from build123d import *

# Parameters (mm, degrees)
SKETCH_1_R          = 15
SKETCH_1_R_2        = 7
EXTRUDE_1_DEPTH     = 2
CUT_EXTRUDE_1_REACH = 23.307
SKETCH_2_R          = 1.1
SKETCH_3_R          = 0.95


with BuildPart() as part:
    # 草图1 → 凸台-拉伸1 (new body)
    with BuildSketch(Plane(origin=(0, 0, 0), x_dir=(1, 0, 0), z_dir=(0, 1, 0))):
        with Locations(Location((0, 0, 0), (0, 0, 270))):
            Circle(SKETCH_1_R)
        with Locations(Location((0, 0, 0), (0, 0, 270))):
            Circle(SKETCH_1_R_2, mode=Mode.SUBTRACT)
    extrude(amount=EXTRUDE_1_DEPTH)

    # 草图2 → 切除-拉伸1 (cut, up to next)
    with BuildSketch(Plane(origin=(0, 2, 0), x_dir=(1, 0, 0), z_dir=(0, 1, 0)), mode=Mode.PRIVATE) as cut_extrude_1_sk1:
        with Locations(Location((12.5, 0, 0), (0, 0, 270))):
            Circle(SKETCH_2_R)
    cut_extrude_1_tool1 = extrude(cut_extrude_1_sk1.sketch, amount=-CUT_EXTRUDE_1_REACH, mode=Mode.PRIVATE) & part.part
    # 草图2 → 切除-拉伸1 (cut, up to next)
    with BuildSketch(Plane(origin=(0, 2, 0), x_dir=(1, 0, 0), z_dir=(0, 1, 0)), mode=Mode.PRIVATE) as cut_extrude_1_sk2:
        with Locations(Location((0, -12.5, 0), (0, 0, 270))):
            Circle(SKETCH_2_R)
    cut_extrude_1_tool2 = extrude(cut_extrude_1_sk2.sketch, amount=-CUT_EXTRUDE_1_REACH, mode=Mode.PRIVATE) & part.part
    # 草图2 → 切除-拉伸1 (cut, up to next)
    with BuildSketch(Plane(origin=(0, 2, 0), x_dir=(1, 0, 0), z_dir=(0, 1, 0)), mode=Mode.PRIVATE) as cut_extrude_1_sk3:
        with Locations(Location((-12.5, 0, 0), (0, 0, 270))):
            Circle(SKETCH_2_R)
    cut_extrude_1_tool3 = extrude(cut_extrude_1_sk3.sketch, amount=-CUT_EXTRUDE_1_REACH, mode=Mode.PRIVATE) & part.part
    # 草图2 → 切除-拉伸1 (cut, up to next)
    with BuildSketch(Plane(origin=(0, 2, 0), x_dir=(1, 0, 0), z_dir=(0, 1, 0)), mode=Mode.PRIVATE) as cut_extrude_1_sk4:
        with Locations(Location((0, 12.5, 0), (0, 0, 270))):
            Circle(SKETCH_2_R)
    cut_extrude_1_tool4 = extrude(cut_extrude_1_sk4.sketch, amount=-CUT_EXTRUDE_1_REACH, mode=Mode.PRIVATE) & part.part
    add(cut_extrude_1_tool1.solids().sort_by_distance((12.5, 2, 0))[0], mode=Mode.SUBTRACT)
    add(cut_extrude_1_tool2.solids().sort_by_distance((0, 2, 12.5))[0], mode=Mode.SUBTRACT)
    add(cut_extrude_1_tool3.solids().sort_by_distance((-12.5, 2, 0))[0], mode=Mode.SUBTRACT)
    add(cut_extrude_1_tool4.solids().sort_by_distance((0, 2, -12.5))[0], mode=Mode.SUBTRACT)

    # 草图3 → 切除-旋转1 (revolve, cut)
    with BuildSketch(Plane.XY, mode=Mode.PRIVATE) as cut_revolve_1_sk:
        with Locations((9.05, 2)):
            Circle(SKETCH_3_R)
    revolve(cut_revolve_1_sk.sketch.rotate(Axis((0, 2, 0), (0, 1, 0)), 90), axis=Axis((0, 2, 0), (0, 1, 0)), mode=Mode.SUBTRACT)


solid = part.part
Work out the finished part from the listing and answer in its coordinate system (mm). Give positions to 0.01 mm unless a question says otherwise; leave off trailing zeros. Write each loop counter-clockwise with the first axis right and the second up, starting at its lowest first coordinate (ties: lowest second). Pieces come first, ordered by that corner, then holes. Notation, with made-up numbers: M 38.5,-36.5 L 67.5,-36.5 A10 ccw 67.5,-19.5 Z; hole C -32,29.5 d11. An arc over 180 degrees is marked long. Answer as CSV lines item,"result".
Q1. A cutting plane is placed at A-A on x = 0. Write down the section's boundary in (y, z), plus the area to 3 significant figures.
A:
outline,"M 0,-15 L 2,-15 L 2,-13.6 L 0,-13.6 Z; M 0,-11.4 L 2,-11.4 L 2,-10 A0.95 cw 2,-8.1 L 2,-7 L 0,-7 Z; M 0,7 L 2,7 L 2,8.1 A0.95 cw 2,10 L 2,11.4 L 0,11.4 Z; M 0,13.6 L 2,13.6 L 2,15 L 0,15 Z"
area,"20.4 mm²"
Q2. A cutting plane is placed at B-B on z = 0. Write down the section's boundary in (x, y), plus the area to 3 significant figures.
A:
outline,"M -15,0 L -13.6,0 L -13.6,2 L -15,2 Z; M -11.4,0 L -7,0 L -7,2 L -8.1,2 A0.95 cw -10,2 L -11.4,2 Z; M 7,0 L 11.4,0 L 11.4,2 L 10,2 A0.95 cw 8.1,2 L 7,2 Z; M 13.6,0 L 15,0 L 15,2 L 13.6,2 Z"
area,"20.4 mm²"
Q3. A cutting plane is placed at D-D on y = 1.7. Write down the section's boundary in (x, z).
A:
outline,"C 0,0 d30; C 0,0 d16.3; hole C -12.5,0 d2.2; hole C 0,0 d19.9; hole C 0,0 d14; hole C 0,-12.5 d2.2; hole C 0,12.5 d2.2; hole C 12.5,0 d2.2"
Q4. A cutting plane is placed at C-C on x = -12.5. Write down the section's boundary in (y, z).
A:
outline,"M 0,-8.29 L 2,-8.29 L 2,-1.1 L 0,-1.1 Z; M 0,1.1 L 2,1.1 L 2,8.29 L 0,8.29 Z"
Q5. Find the intervals of material crossed by probe 1 along X at (y, z) = (0.55, 0); probe 2 along X at (y, z) = (1.35, 0); probe 3 along X at (y, z) = (1.65, 6), in increasing order. Write a range as [from, to].
A:
probe 1,"x = [-15, -13.6], [-11.4, -7], [7, 11.4], [13.6, 15]"
probe 2,"x = [-15, -13.6], [-11.4, -9.74], [-8.36, -7], [7, 8.36], [9.74, 11.4], [13.6, 15]"
probe 3,"x = [-13.75, -7.92], [-5.54, -3.61], [3.61, 5.54], [7.92, 13.75]"
